from build123d import *

# Parameters (mm, degrees)
SKETCH1_R           = 45
SKETCH1_R_2         = 42
BOSS_EXTRUDE1_DEPTH = 20
SKETCH2_R           = 51
SKETCH2_R_2         = 1.5
SKETCH2_R_3         = 45
BOSS_EXTRUDE2_DEPTH = 5
BOSS_EXTRUDE3_START = -20
SKETCH3_R           = 42
SKETCH3_R_2         = 41.5
BOSS_EXTRUDE3_DEPTH = 20
SKETCH5_R           = 1.5
BOSS_EXTRUDE4_DEPTH = 1.5


with BuildPart() as part:
    # Sketch1 → Boss-Extrude1 (new body)
    with BuildSketch(Plane(origin=(0, 0, 0), x_dir=(1, 0, 0), z_dir=(0, 1, 0))):
        with Locations(Location((0, 0, 0), (0, 0, 270))):
            Circle(SKETCH1_R)
        with Locations(Location((0, 0, 0), (0, 0, 270))):
            Circle(SKETCH1_R_2, mode=Mode.SUBTRACT)
    extrude(amount=BOSS_EXTRUDE1_DEPTH)

    # Sketch2 → Boss-Extrude2 (add)
    with BuildSketch(Plane.XZ):
        with Locations(Location((0, 0, 0), (0, 0, 270))):
            Circle(SKETCH2_R)
        with Locations(Location((0, -48, 0), (0, 0, 270))):
            Circle(SKETCH2_R_2, mode=Mode.SUBTRACT)
        with Locations(Location((-48, 0, 0), (0, 0, 270))):
            Circle(SKETCH2_R_2, mode=Mode.SUBTRACT)
        with Locations(Location((0, 0, 0), (0, 0, 270))):
            Circle(SKETCH2_R_3, mode=Mode.SUBTRACT)
        with BuildLine():
            ThreePointArc((49.5, 0), (48, -1.5), (46.5, 0))
            ThreePointArc((46.5, 0), (48, 1.5), (49.5, 0))
        make_face(mode=Mode.SUBTRACT)
        with Locations(Location((0, 48, 0), (0, 0, 270))):
            Circle(SKETCH2_R_2, mode=Mode.SUBTRACT)
    extrude(amount=-BOSS_EXTRUDE2_DEPTH)

    # Sketch3 → Boss-Extrude3 (add)
    with BuildSketch(Plane(origin=(0, 20, 0), x_dir=(1, 0, 0), z_dir=(0, 1, 0)).offset(BOSS_EXTRUDE3_START)):
        Circle(SKETCH3_R)
        with Locations(Location((0, 0, 0), (0, 0, 270))):
            Circle(SKETCH3_R_2, mode=Mode.SUBTRACT)
    extrude(amount=BOSS_EXTRUDE3_DEPTH)

    # Sketch5 → Boss-Extrude4 (add)
    # profile 1 of 4: a face of its own
    with BuildSketch(Plane.XZ):
        with BuildLine():
            Line((35.5, 3), (42.194384288, 3))
            Line((42.194384288, 3), (42.194384288, -3))
            Line((42.194384288, -3), (35.5, -3))
            ThreePointArc((35.5, -3), (32.5, 0), (35.5, 3))
        make_face()
        with Locations(Location((35.5, 0, 0), (0, 0, 270))):
            Circle(SKETCH5_R, mode=Mode.SUBTRACT)
    # profile 2 of 4: a face of its own
    with BuildSketch(Plane.XZ):
        with BuildLine():
            Line((-3, 35.5), (-3, 42.194384288))
            Line((-3, 42.194384288), (3, 42.194384288))
            Line((3, 42.194384288), (3, 35.5))
            ThreePointArc((3, 35.5), (0, 32.5), (-3, 35.5))
        make_face()
        with Locations(Location((0, 35.5, 0), (0, 0, 270))):
            Circle(SKETCH5_R, mode=Mode.SUBTRACT)
    # profile 3 of 4: a face of its own
    with BuildSketch(Plane.XZ):
        with BuildLine():
            Line((3, -35.5), (3, -42.194384288))
            Line((3, -42.194384288), (-3, -42.194384288))
            Line((-3, -42.194384288), (-3, -35.5))
            ThreePointArc((-3, -35.5), (0, -32.5), (3, -35.5))
        make_face()
        with Locations(Location((0, -35.5, 0), (0, 0, 270))):
            Circle(SKETCH5_R, mode=Mode.SUBTRACT)
    # profile 4 of 4: a face of its own
    with BuildSketch(Plane.XZ):
        with BuildLine():
            Line((-35.5, -3), (-42.194384288, -3))
            Line((-42.194384288, -3), (-42.194384288, 3))
            Line((-42.194384288, 3), (-35.5, 3))
            ThreePointArc((-35.5, 3), (-32.5, 0), (-35.5, -3))
        make_face()
        with Locations(Location((-35.5, 0, 0), (0, 0, 270))):
            Circle(SKETCH5_R, mode=Mode.SUBTRACT)
    extrude(amount=-BOSS_EXTRUDE4_DEPTH)


solid = part.part
Design review of the part built by this model. Coordinates are the model's own, in mm. A direction names the side the tool comes from. Give positions to 0.01 mm unless a question says otherwise; leave off trailing zeros. Write each loop counter-clockwise with the first axis right and the second up, starting at its lowest first coordinate (ties: lowest second). Pieces come first, ordered by that corner, then holes. Notation, with made-up numbers: M -10,53 L -4,53 A25 cw -4,80 Z; hole C 78,70 d5. An arc over 180 degrees is marked long. Answer as a JSON object with one key per item and string values. Group by question number.
1) Clearance check with flat-ended pins moving along their axes: pin 1 Ø1.5 at (y, z) = (13.5, 36) entering from -X; pin 2 Ø4 at (x, y) = (26.5, 11.5) entering from +Z; pin 3 Ø5 at (y, z) = (14.5, -9) entering from -X. State where each tip first meets the part, or that it passes through.
2) We need section B-B (z = 48). Give the boundary of the cut face in (x, y), and give its area (3 significant figures).
3) For line 1 along X through (y, z) = (10.75, 0); line 2 along X through (y, z) = (1.25, -35.5), list the stretches that pass through material, from the lowest coordinate up.
4) Tool access review of faces 4 (the face through (-38, 1.5, 0)), 5 (the face through (32.5, 0.7, -0.1)): name each direction out of +Z, -Z, +X, -X, +Y, -Y from which nothing blocks a thin tool from reaching the whole face with its end or side.
5) We need section D-D (y = 9.5). Give the boundary of the cut face in (x, z).
6) We need section C-C (x = 48). Give the boundary of the cut face in (y, z).
7) We need section A-A (x = 0). Count the separate pieces of the cut face and the enclosed holes in it, and give its area (3 significant figures).
8) Mouldability with a two-part tool opening along X and no side actions: class faces 1 (the face through (13, 20, 40)), 2 (the face through (0.07, 2.46, -46.5)), 3 (the face through (-17.235, 12.395, 41.569)) as released by +X, released by -X, zero draft, split by the parting line, or undercut.
Answer key:
{
 "1": {"pin 1": "stops at x = -27.97", "pin 2": "stops at z = 37.75", "pin 3": "stops at x = -44.53"},
 "2": {"outline": "M -17.23,0 L -1.5,0 L -1.5,5 L -17.23,5 Z; M 1.5,0 L 17.23,0 L 17.23,5 L 1.5,5 Z", "area": "157 mm²"},
 "3": {"line 1": "x = -45 to -41.5, 41.5 to 45", "line 2": "x = -36.62 to -21.49, -3 to -1.5, 1.5 to 3, 21.49 to 36.62"},
 "4": {"face 4": "+Y", "face 5": "+Y, -Y"},
 "5": {"outline": "C 0,0 d90; hole C 0,0 d83"},
 "6": {"outline": "M 0,-17.23 L 5,-17.23 L 5,-1.5 L 0,-1.5 Z; M 0,1.5 L 5,1.5 L 5,17.23 L 0,17.23 Z"},
 "7": {"separate pieces": "6", "enclosed holes": "0", "area": "188 mm²"},
 "8": {"face 1": "zero draft", "face 2": "undercut", "face 3": "split by the parting line"}
}
